from build123d import *

# Parameters (mm, degrees)
SZKIC1_R                    = 0.75
DODANIE_WYCI_GNI_CIE1_DEPTH = 9
ZAOKR_GLENIE1_R             = 2
ZAOKR_GLENIE3_R             = 1
SZKIC2_R                    = 1.7
WYTNIJ_WYCI_GNI_CIE1_DEPTH  = 27647.561311418
SZKIC3_W                    = 13.077407628
SZKIC3_H                    = 7
SZKIC3_W_2                  = 12.422592372
WYTNIJ_WYCI_GNI_CIE2_DEPTH  = 27647.561311418
SZKIC4_W                    = 7.2
SZKIC4_H                    = 12.770373744
WYTNIJ_WYCI_GNI_CIE3_DEPTH  = 17269.61853488
ZAOKR_GLENIE4_R             = 2
ZAOKR_GLENIE5_R             = 1
ZAOKR_GLENIE7_R             = 0.2
DODANIE_WYCI_GNI_CIE3_DEPTH = 7.2


with BuildPart() as part:
    # Szkic1 → Dodanie-wyciągnięcie1 (new body)
    with BuildSketch(Plane.XY):
        Polygon((-27646.558741393, -28.902320952), (-27646.558741393, -33.902320952), (-27597.758741393, -33.902320952), (-27589.47352106, -23.517649804), (-27592.522131216, -21.085371835), (-27598.758741393, -28.902320952), (-27634.258741393, -28.902320952), (-27634.258741393, -23.902320952), (-27638.758741393, -23.902320952), (-27638.758741393, -28.902320952), align=None)
        with Locations((-27600.758741393, -31.402320952)):
            Circle(SZKIC1_R, mode=Mode.SUBTRACT)
    extrude(amount=DODANIE_WYCI_GNI_CIE1_DEPTH)

    # Zaokrąglenie1
    zaokr_glenie1_edges = [part.edges().sort_by_distance(p)[0] for p in [
        (-27638.758741393, -23.902320952, 4.5),
        (-27634.258741393, -23.902320952, 4.5),
        (-27646.558741393, -33.902320952, 4.5),
        (-27646.558741393, -28.902320952, 4.5),
    ]]
    fillet(zaokr_glenie1_edges, radius=ZAOKR_GLENIE1_R)

    # Zaokrąglenie3
    zaokr_glenie3_edges = [part.edges().sort_by_distance(p)[0] for p in [
        (-27597.758741393, -33.902320952, 4.5),
    ]]
    fillet(zaokr_glenie3_edges, radius=ZAOKR_GLENIE3_R)

    # Szkic2 → Wytnij-wyciągnięcie1 (cut, through all)
    with BuildSketch(Plane(origin=(0, -28.902320952, 0), x_dir=(1, 0, 0), z_dir=(0, 1, 0))):
        with Locations(Location((-27641.658741393, -4.5, 0), (0, 0, 180))):
            Circle(SZKIC2_R)
    extrude(amount=-WYTNIJ_WYCI_GNI_CIE1_DEPTH, mode=Mode.SUBTRACT)

    # Szkic3 → Wytnij-wyciągnięcie2 (cut, through all)
    with BuildSketch(Plane(origin=(0, -28.902320952, 0), x_dir=(1, 0, 0), z_dir=(0, 1, 0))):
        with Locations((-27609.297445207, -4.5)):
            Rectangle(SZKIC3_W, SZKIC3_H)
        with Locations((-27625.047445207, -4.5)):
            Rectangle(SZKIC3_W_2, SZKIC3_H)
    extrude(amount=-WYTNIJ_WYCI_GNI_CIE2_DEPTH, mode=Mode.SUBTRACT)

    # Szkic4 → Wytnij-wyciągnięcie3 (cut, through all)
    with BuildSketch(Plane(origin=(-16850.04669364, 13443.502203136, 0), x_dir=(0, 0, 1), z_dir=(-0.7816949117558672, 0.6236610176490005, 0))):
        with Locations((4.6, -17228.477572842)):
            Rectangle(SZKIC4_W, SZKIC4_H)
    extrude(amount=-WYTNIJ_WYCI_GNI_CIE3_DEPTH, mode=Mode.SUBTRACT)

    # Zaokrąglenie4
    # the kernel refuses this fillet: 2 mm, written as the material it takes off along each edge
    with BuildSketch(Plane(origin=(-27589.47352106, -23.517649804, -5), x_dir=(-0.6236610176488676, -0.7816949117559733, 0), z_dir=(0, 0, 1)), Plane(origin=(-27592.522131216, -21.085371835, -5), x_dir=(0.78169491175572, -0.623661017649185, 0), z_dir=(0, 0, 1))) as zaokr_glenie4_piece_1:
        with BuildLine():
            CenterArc((ZAOKR_GLENIE4_R, -ZAOKR_GLENIE4_R), ZAOKR_GLENIE4_R, 90, 90)
            Line((0, -ZAOKR_GLENIE4_R), (0, 0))
            Line((0, 0), (ZAOKR_GLENIE4_R, 0))
        make_face()
    extrude(amount=11, mode=Mode.SUBTRACT)
    with BuildSketch(Plane(origin=(-27589.47352106, -23.517649804, 3.2), x_dir=(-0.6236610176488676, -0.7816949117559733, 0), z_dir=(0, 0, 1)), Plane(origin=(-27592.522131216, -21.085371835, 3.2), x_dir=(0.78169491175572, -0.623661017649185, 0), z_dir=(0, 0, 1))) as zaokr_glenie4_piece_2:
        with BuildLine():
            CenterArc((ZAOKR_GLENIE4_R, -ZAOKR_GLENIE4_R), ZAOKR_GLENIE4_R, 90, 90)
            Line((0, -ZAOKR_GLENIE4_R), (0, 0))
            Line((0, 0), (ZAOKR_GLENIE4_R, 0))
        make_face()
    extrude(amount=10.8, mode=Mode.SUBTRACT)

    # Zaokrąglenie5
    zaokr_glenie5_edges = [part.edges().sort_by_distance(p)[0] for p in [
        (-27639.958741393, -33.902320952, 4.5),
    ]]
    fillet(zaokr_glenie5_edges, radius=ZAOKR_GLENIE5_R)

    # Zaokrąglenie7
    zaokr_glenie7_edges = [part.edges().sort_by_distance(p)[0] for p in [
        (-27601.508741393, -31.402320952, 0),
        (-27601.508741393, -31.402320952, 9),
    ]]
    fillet(zaokr_glenie7_edges, radius=ZAOKR_GLENIE7_R)

    # Szkic6 → Dodanie-wyciągnięcie3 (add)
    with BuildSketch(Plane.XY.offset(1)):
        with BuildLine():
            ThreePointArc((-27591.372412611, -22.771016391), (-27592.075090576, -22.850033338), (-27591.996073629, -23.552711303))
            Line((-27591.996073629, -23.552711303), (-27591.372412611, -22.771016391))
        make_face()
        with BuildLine():
            Line((-27591.372412611, -22.771016391), (-27591.996073629, -23.552711303))
            ThreePointArc((-27591.996073629, -23.552711303), (-27591.467350583, -23.612372035), (-27591.18424312, -23.161863847))
            ThreePointArc((-27591.18424312, -23.161863847), (-27591.233734932, -22.944971309), (-27591.372412611, -22.771016391))
        make_face()
    extrude(amount=DODANIE_WYCI_GNI_CIE3_DEPTH)


solid = part.part
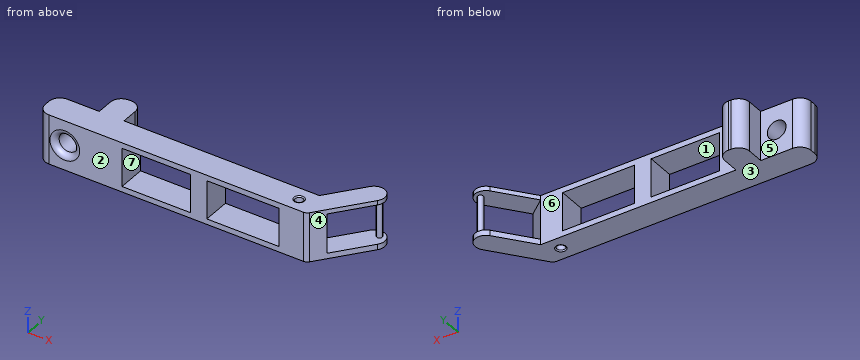
The listing builds one solid part. Answer for the finished solid, in the listing's coordinates (mm). Face numbers are marked on the shaded views. A direction names the side the tool comes from. Round coordinates to 2 decimals unless told otherwise and drop trailing zeros. Order: outer loops, then holes, each group sorted by start corner. A loop starts at its lowest first (then second) coordinate and runs counter-clockwise, first axis right, second up. Notation, with made-up numbers: M 42.5,78 L 79.5,78 A15 ccw 79.5,83 Z; hole C 30,30.25 d4. An arc over 180 degrees is marked long. Answer in a Markdown table with one row per item. Add a question column.
1) Consider line 1 along Z through (x, y) = (-27622.5, -32.25); line 2 along X through (y, z) = (-33.5, 2.5); line 3 along X through (y, z) = (-31.75, 6.5). Determine where each line is inside the solid, lowest interval first. Write a range as from..to.
2) Which of the six approach directions +Z, -Z, +X, -X, +Y, -Y give full straight-line access (tool end or side, diameter ignored) to the marked faces 4, 5, 6 and 7?
3) Determine the mould class of the marked faces 1, 2 and 3 for opening direction Z: pulls with the +Z half, pulls with the -Z half, needs draft (parallel to the pull), parting line crosses it, or undercut.
4) The part is cut by section A-A on x = -27615. Determine the outline of the cut face in (y, z).
5) The part is cut by section C-C on y = -27.5. Determine the outline of the cut face in (x, z).
6) Flat-ended cylindrical pins translate along their axes: pin 1 Ø4 at (x, z) = (-27641.66, 4.5) entering from +Y; pin 2 Ø3 at (y, z) = (-24, 6) entering from -X; pin 3 Ø3.5 at (y, z) = (-28, 5.5) entering from +X. Find the tip coordinate at first contact, or state that the pin passes through.
7) The part is cut by section D-D on y = -29.75. Determine the outline of the cut face in (x, z), plus the area to 3 significant figures.
8) The part is cut by section B-B on z = 4.5. Count the separate pieces of the cut face and the enclosed holes in it, plus the area to 3 significant figures.
Findings below:
| question | item | result |
|---|---|---|
| 1 | line 1 | z = 0..1, 8..9 |
| 1 | line 2 | x = -27645.76..-27631.26, -27618.84..-27615.84, -27602.76..-27597.44 |
| 1 | line 3 | x = -27646.56..-27631.26, -27618.84..-27615.84, -27602.76..-27601.42, -27600.09..-27596.04 |
| 2 | face 4 | +Z, -Z, +X, -Y |
| 2 | face 5 | +Z, -Z, -X, +Y |
| 2 | face 6 | +Z, -Z, +Y |
| 2 | face 7 | +Y, -Y |
| 3 | face 1 | undercut |
| 3 | face 2 | needs draft |
| 3 | face 3 | pulls with the -Z half |
| 4 | outline | M -33.9,0 L -28.9,0 L -28.9,1 L -33.9,1 Z; M -33.9,8 L -28.9,8 L -28.9,9 L -33.9,9 Z |
| 5 | outline | M -27638.76,0 L -27634.26,0 L -27634.26,9 L -27638.76,9 Z; M -27597.64,0 L -27592.65,0 L -27592.65,1 L -27597.64,1 Z; M -27597.64,8.2 L -27592.65,8.2 L -27592.65,9 L -27597.64,9 Z |
| 6 | pin 1 | stops at y = -28.9 |
| 6 | pin 2 | stops at x = -27638.72 |
| 6 | pin 3 | stops at x = -27597.7 |
| 7 | outline | M -27646.19,0 L -27594.45,0 L -27594.45,1 L -27597.7,1 L -27597.7,8.2 L -27594.45,8.2 L -27594.45,9 L -27646.19,9 Z; hole C -27641.66,4.5 d3.4; hole M -27631.26,1 L -27618.84,1 L -27618.84,8 L -27631.26,8 Z; hole M -27615.84,1 L -27602.76,1 L -27602.76,8 L -27615.84,8 Z |
| 7 | area | 255 mm² |
| 8 | separate pieces | 5 |
| 8 | enclosed holes | 1 |
| 8 | area | 121 mm² |
